Here's the drawing with two shaded views (mm, measured from the low corner). I have some questions. A direction names the side the tool comes from. Coordinates: 2 decimals unless noted, no trailing zeros. Order: outer loops, then holes, each group sorted by start corner. A loop starts at its lowest first (then second) coordinate and runs counter-clockwise, first axis right, second up. Notation, with made-up numbers: (9.5, -28.75) -> (63.5, -28.75) arc R18 ccw to (63.5, -0.75) -> close; hole circle Ø3 at (14, -12.5). An arc over 180 degrees is marked (long way). Write item = value, one per line.
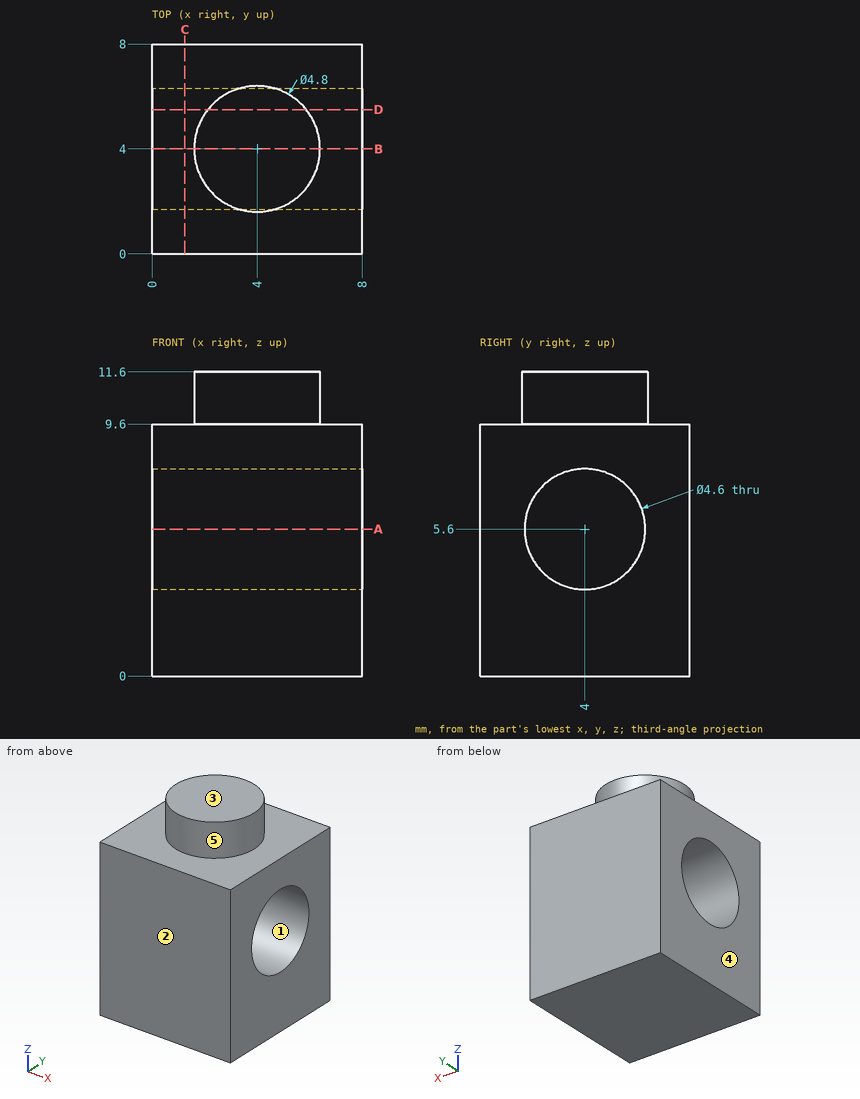
Item 1: I want a section at A-A, the plane z = 5.6. Please give me the cut outline in (x, y).
A:
outline = (0, 0) -> (8, 0) -> (8, 1.7) -> (0, 1.7) -> close; (0, 6.3) -> (8, 6.3) -> (8, 8) -> (0, 8) -> close
Item 2: I want a section at D-D, the plane y = 5.5. Please give me the cut outline in (x, z).
A:
outline = (0, 0) -> (8, 0) -> (8, 3.86) -> (0, 3.86) -> close; (0, 7.34) -> (8, 7.34) -> (8, 9.6) -> (5.87, 9.6) -> (5.87, 11.6) -> (2.13, 11.6) -> (2.13, 9.6) -> (0, 9.6) -> close
Item 3: I want a section at B-B, the plane y = 4. Please give me the cut outline in (x, z), plus the area to 3 significant figures.
A:
outline = (0, 0) -> (8, 0) -> (8, 3.3) -> (0, 3.3) -> close; (0, 7.9) -> (8, 7.9) -> (8, 9.6) -> (6.4, 9.6) -> (6.4, 11.6) -> (1.6, 11.6) -> (1.6, 9.6) -> (0, 9.6) -> close
area = 49.6 mm2
Item 4: I want a section at C-C, the plane x = 1.25. Please give me the cut outline in (y, z).
A:
outline = (0, 0) -> (8, 0) -> (8, 9.6) -> (0, 9.6) -> close; hole circle Ø4.6 at (4, 5.6)
Item 5: For the marked faces 4 and 5, which set-ups out of +Z, -Z, +X, -X, +Y, -Y let a thin tool reach every point of the face, with its end or its side?
A:
face_4 = +Z, -Z, -X, +Y, -Y
face_5 = +Z
Item 6: If I drill on probe 1 along Z at (x, y) = (6.25, 4); probe 2 along Z at (x, y) = (1.5, 4); probe 3 along Y at (x, z) = (5, 3.75), over which ranges is the centre line in solid material (lowest first)?
A:
probe_1 = 0 to 3.3, 7.9 to 11.6
probe_2 = 0 to 3.3, 7.9 to 9.6
probe_3 = 0 to 2.63, 5.37 to 8
Item 7: If we mould it in two halves opening along Z, with no side actions, what happens to the marked faces 1, 2 and 3? For each: pulls with the +Z half, pulls with the -Z half, needs draft (parallel to the pull), parting line crosses it, or undercut.
A:
face_1 = undercut
face_2 = needs draft
face_3 = pulls with the +Z half
Item 8: I'm going to push flat-ended pins straight in: P1, Ø2, axis at y = 6.5, z = 4.5, coming from the -X side; P2, Ø4, axis at y = 4, z = 5.6, coming from the +X side. Where does each tip first touch, or does it pass through?
A:
P1 = 0
P2 = through
